Check sheet for the drawn part. Datum: minimum x, y, z corner. Units: mm. Coordinates: 2 decimals unless noted, no trailing zeros. Write each loop counter-clockwise with the first axis right and the second up, starting at its lowest first coordinate (ties: lowest second). Pieces come first, ordered by that corner, then holes. Notation, with made-up numbers: (68, 28) -> (97, 28) arc R16 cw to (97, 58) -> close; hole circle Ø9 at (-17, 30). An arc over 180 degrees is marked (long way). Write item = value, one per line. Start each with the question number.
(1) Section check A-A (x = 45). Record the cut outline in (y, z), plus the area to 3 significant figures.
(2) Section check B-B (z = 4.5). Record the cut outline in (x, y), plus the area to 3 significant figures.
(3) Mould release check, pull along Y, two halves, no side actions. Record for the marked faces 1, 2 and 3: released by +Y, released by -Y, zero draft, split by the parting line, or undercut.
(4) Material ranges on probe 1 along X at (y, z) = (3.25, 5.25); probe 2 along Y at (x, z) = (10, 4.5); probe 3 along Y at (x, z) = (9.5, 2), recorded low to high. Write a range as [from, to].
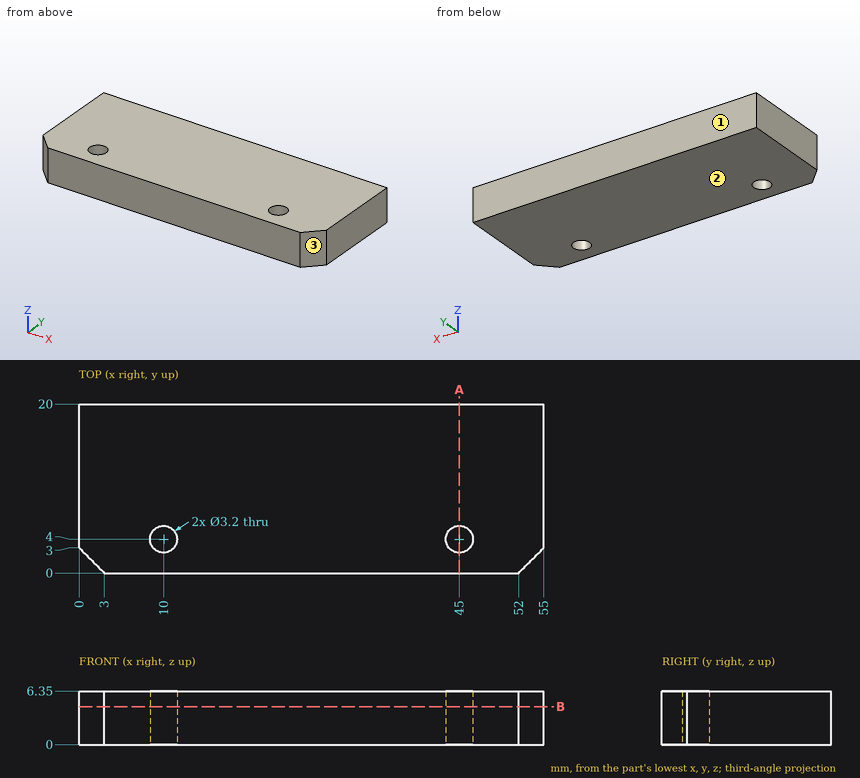
Response:
q1.outline = (0, 0) -> (2.4, 0) -> (2.4, 6.35) -> (0, 6.35) -> close; (5.6, 0) -> (20, 0) -> (20, 6.35) -> (5.6, 6.35) -> close
q1.area = 107 mm2
q2.outline = (0, 3) -> (3, 0) -> (52, 0) -> (55, 3) -> (55, 20) -> (0, 20) -> close; hole circle Ø3.2 at (10, 4); hole circle Ø3.2 at (45, 4)
q2.area = 1,070 mm2
q3.face_1 = released by +Y
q3.face_2 = zero draft
q3.face_3 = released by -Y
q4.probe_1 = [0, 8.59], [11.41, 43.59], [46.41, 55]
q4.probe_2 = [0, 2.4], [5.6, 20]
q4.probe_3 = [0, 2.48], [5.52, 20]
